```python
from build123d import *

# Parameters (mm, degrees)
SKETCH_1_R             = 7.5
SKETCH_1_R_2           = 2
EXTRUDE_1_DEPTH        = 5
EXTRUDE_START          = -5
EXTRUDE_2_DEPTH        = 5
SKETCH_3_R             = 1
CUT_EXTRUDE_1_DEPTH    = 5
EXTRUDE_3_DEPTH        = 5
FILLET_1_R             = 10
SKETCH_11_R            = 5
CUT_EXTRUDE_4_DEPTH    = 2.5
SKETCH_12_R            = 1
CUT_EXTRUDE_5_DEPTH    = 19.45893317
HOLE_WIZARD_M3_1_D     = 2.5
HOLE_WIZARD_M3_1_DEPTH = 8.5
HOLE_WIZARD_M3_1_TIP   = 0.751075774


with BuildPart() as part:
    # ｽｹｯﾁ1 → ﾎﾞｽ - 押し出し1 (new body)
    with BuildSketch(Plane.XY):
        Circle(SKETCH_1_R)
        Circle(SKETCH_1_R_2, mode=Mode.SUBTRACT)
    extrude(amount=EXTRUDE_1_DEPTH)

    # ｽｹｯﾁ2 → ﾎﾞｽ - 押し出し2 (add)
    with BuildSketch(Plane.XY.offset(5).offset(EXTRUDE_START)):
        with BuildLine():
            Line((-7.5, 0), (-7.5, 15))
            Line((-7.5, 15), (7.5, 15))
            Line((7.5, 15), (7.5, 0))
            ThreePointArc((7.5, 0), (0, 7.5), (-7.5, 0))
        make_face()
    extrude(amount=EXTRUDE_2_DEPTH)

    # ｽｹｯﾁ3 → ｶｯﾄ - 押し出し1 (cut)
    with BuildSketch(Plane(origin=(0, 15, 0), x_dir=(1, 0, 0), z_dir=(0, 1, 0))):
        with Locations(Location((-4.5, -2.5, 0), (0, 0, 270))):
            Circle(SKETCH_3_R)
        with Locations(Location((4.5, -2.5, 0), (0, 0, 90))):
            Circle(SKETCH_3_R)
    extrude(amount=-CUT_EXTRUDE_1_DEPTH, mode=Mode.SUBTRACT)

    # ｽｹｯﾁ4 → ﾎﾞｽ - 押し出し3 (add)
    with BuildSketch(Plane.XY.offset(5).offset(EXTRUDE_START)):
        with BuildLine():
            Line((-7.5, 15), (-10, 7.5))
            Line((-10, 7.5), (-7.2, -2.1))
            ThreePointArc((-7.2, -2.1), (-7.424621202, -1.060660172), (-7.5, 0))
            Line((-7.5, 0), (-7.5, 15))
        make_face()
        with BuildLine():
            Line((7.5, 0), (7.5, 15))
            Line((7.5, 15), (10, 7.5))
            Line((10, 7.5), (7.2, -2.1))
            ThreePointArc((7.2, -2.1), (7.424621202, -1.060660172), (7.5, 0))
        make_face()
    extrude(amount=EXTRUDE_3_DEPTH)

    # ﾌｨﾚｯﾄ1
    fillet_1_edges = [part.edges().sort_by_distance(p)[0] for p in [
        (-10, 7.5, 2.5),
        (10, 7.5, 2.5),
    ]]
    fillet(fillet_1_edges, radius=FILLET_1_R)

    # ｽｹｯﾁ11 → ｶｯﾄ - 押し出し4 (cut)
    with BuildSketch(Plane.XY.offset(5)):
        Circle(SKETCH_11_R)
    extrude(amount=-CUT_EXTRUDE_4_DEPTH, mode=Mode.SUBTRACT)

    # ｽｹｯﾁ12 → ｶｯﾄ - 押し出し5 (cut, through all)
    with BuildSketch(Plane(origin=(0, 0, 0), x_dir=(-1, 0, 0), z_dir=(0, 0, -1))):
        with Locations((-4.5, 15.8)):
            Circle(SKETCH_12_R)
        with Locations((4.5, 15.8)):
            Circle(SKETCH_12_R)
    extrude(amount=-CUT_EXTRUDE_5_DEPTH, mode=Mode.SUBTRACT)

    # M3 ねじ穴1
    with Locations(Plane(origin=(0, 15, 0), x_dir=(1, 0, 0), z_dir=(0, 1, 0))):
        with Locations((-4.5, -2.5), (4.5, -2.5)):
            Hole(HOLE_WIZARD_M3_1_D / 2, depth=HOLE_WIZARD_M3_1_DEPTH)
            with Locations((0, 0, -(HOLE_WIZARD_M3_1_DEPTH + HOLE_WIZARD_M3_1_TIP / 2))):  # 118° drill point
                Cone(0, HOLE_WIZARD_M3_1_D / 2, HOLE_WIZARD_M3_1_TIP, mode=Mode.SUBTRACT)


solid = part.part
```
Work out the finished part from the listing and answer in its coordinate system (mm). A direction names the side the tool comes from. Round coordinates to 2 decimals unless told otherwise and drop trailing zeros. Write each loop counter-clockwise with the first axis right and the second up, starting at its lowest first coordinate (ties: lowest second). Pieces come first, ordered by that corner, then holes. Notation, with made-up numbers: (51, 35) - (92, 35) arc R12 ccw to (92, 57) - close; hole circle Ø6 at (75.5, -1.75). An arc over 180 degrees is marked (long way). Return JSON: item names as keys, results as strings. Group by question number.
Q1. The part is cut by section A-A on x = 0. Write down the section's boundary in (y, z).
Q2. The part is cut by section D-D on x = 3. Write down the section's boundary in (y, z).
Q3. The mould has two halves that part along X. Classify faces 3 (the cylindrical face through (5.421, 10.691, 1.655)), 4 (the cylindrical face through (-4.34, 10.69, 1.26)), 5 (the flat face through (-6, 15, 2)), 6 (the flat face through (-8.246, 12.763, 2.465)): released by +X, released by -X, zero draft, split by the parting line, or undercut.
Q4. Find the intervals of material crossed by L1, parallel to Y at x = 0, z = 0.8; L2, parallel to Y at x = 0, z = 3.85; L3, parallel to X at y = 8, z = 3.6, in increasing order.
Q5. The part is cut by section B-B on y = 12.75. Write down the section's boundary in (x, z), then the cut area to 3 significant figures.
Q6. For faces 1 (the conical face through (-4.66, 5.88, 2.35)), 2 (the flat face through (-0.1, -2.2, 2.5)), determine the directions among +Z, -Z, +X, -X, +Y, -Y from which every point of the face is accessible in a straight line to the end or side of a thin tool.
Q7. Each of these flat-tipped pins is pushed along its axis until it touches: pin 1 Ø3.5 at (x, y) = (0, 0) entering from -Z; pin 2 Ø2 at (y, z) = (-5, 4.5) entering from -X; pin 3 Ø3 at (x, z) = (-4.5, 2.5) entering from -Y; pin 4 Ø1.5 at (y, z) = (2, 0.5) entering from +X. Where does it stop, or does it pass through?
Q8. The part is cut by section C-C on y = 0. Write down the section's boundary in (x, z).
Solved:
{
 "1": {"outline": "(-7.5, 0) - (-2, 0) - (-2, 2.5) - (-5, 2.5) - (-5, 5) - (-7.5, 5) - close; (2, 0) - (15, 0) - (15, 5) - (5, 5) - (5, 2.5) - (2, 2.5) - close"},
 "2": {"outline": "(-6.87, 0) - (15, 0) - (15, 5) - (4, 5) - (4, 2.5) - (-4, 2.5) - (-4, 5) - (-6.87, 5) - close"},
 "3": {"face 3": "undercut", "face 4": "undercut", "face 5": "zero draft", "face 6": "released by -X"},
 "4": {"L1": "-7.5 to -2, 2 to 15", "L2": "-7.5 to -5, 5 to 15", "L3": "-9.5 to -5.09, -3.91 to 3.91, 5.09 to 9.5"},
 "5": {"outline": "(-8.25, 0) - (8.25, 0) - (8.25, 5) - (-8.25, 5) - close; hole circle Ø2.5 at (-4.5, 2.5); hole circle Ø2.5 at (4.5, 2.5)", "area": "72.7 mm²"},
 "6": {"face 1": "+Y", "face 2": "+Z"},
 "7": {"pin 1": "through", "pin 2": "x = -6.34", "pin 3": "y = -6.87", "pin 4": "x = 8.61"},
 "8": {"outline": "(-7.81, 0) - (-2, 0) - (-2, 2.5) - (-5, 2.5) - (-5, 5) - (-7.81, 5) - close; (2, 0) - (7.81, 0) - (7.81, 5) - (5, 5) - (5, 2.5) - (2, 2.5) - close"}
}
